```python
from build123d import *

# Parameters (mm, degrees)
SKETCH_1_R                  = 3
EXTRUDE_1_DEPTH             = 9
SKETCH_2_R                  = 6
EXTRUDE_2_DEPTH             = 1.2
DOME_1_FACE_RADIUS          = 6
DOME_1_HEIGHT               = 3
MIRROR_1_COPY_1_FACE_RADIUS = 6
MIRROR_1_COPY_1_HEIGHT      = 3


with BuildPart() as part:
    # Эскиз1 → Бобышка-Вытянуть1 (new, symmetric)
    with BuildSketch(Plane(origin=(0, 0, 0), x_dir=(1, 0, 0), z_dir=(0, 1, 0))):
        with Locations(Location((0, 0, 0), (0, 0, 270))):
            Circle(SKETCH_1_R)
    extrude(amount=EXTRUDE_1_DEPTH, both=True)

    # Эскиз2 → Бобышка-Вытянуть2 (add)
    with BuildSketch(Plane(origin=(0, 9, 0), x_dir=(1, 0, 0), z_dir=(0, 1, 0))):
        with Locations(Location((0, 0, 0), (0, 0, 270))):
            Circle(SKETCH_2_R)
    extrude_2 = extrude(amount=EXTRUDE_2_DEPTH)

    # Купол1: a dome of height H over a round flat face of radius A is a cap of a sphere of radius (A * A + H * H) / (2 * H)
    dome_1_r = (DOME_1_FACE_RADIUS * DOME_1_FACE_RADIUS + DOME_1_HEIGHT * DOME_1_HEIGHT) / (2 * DOME_1_HEIGHT)
    dome_1_base = Plane((0, 10.2, 0), z_dir=(0, 1, 0))
    with Locations(dome_1_base.offset(DOME_1_HEIGHT - dome_1_r)):
        dome_1_ball = Sphere(dome_1_r, mode=Mode.PRIVATE)
    add(split(dome_1_ball, bisect_by=dome_1_base, keep=Keep.TOP, mode=Mode.PRIVATE))

    # Зеркальное отражение1: Бобышка-Вытянуть2 across plane
    add(extrude_2.mirror(Plane.ZX))

    # Зеркальное отражение1 copy 1: a dome of height H over a round flat face of radius A is a cap of a sphere of radius (A * A + H * H) / (2 * H)
    mirror_1_copy_1_r = (MIRROR_1_COPY_1_FACE_RADIUS * MIRROR_1_COPY_1_FACE_RADIUS + MIRROR_1_COPY_1_HEIGHT * MIRROR_1_COPY_1_HEIGHT) / (2 * MIRROR_1_COPY_1_HEIGHT)
    mirror_1_copy_1_base = Plane((0, -10.2, 0), z_dir=(0, -1, 0))
    with Locations(mirror_1_copy_1_base.offset(MIRROR_1_COPY_1_HEIGHT - mirror_1_copy_1_r)):
        mirror_1_copy_1_ball = Sphere(mirror_1_copy_1_r, mode=Mode.PRIVATE)
    add(split(mirror_1_copy_1_ball, bisect_by=mirror_1_copy_1_base, keep=Keep.TOP, mode=Mode.PRIVATE))


solid = part.part
```
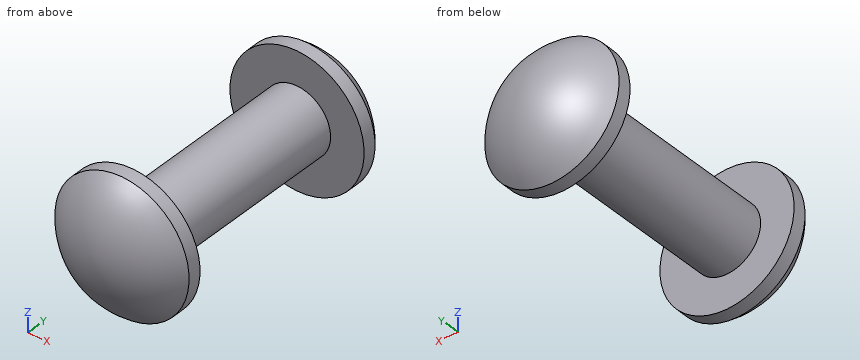
Work out the finished part from the listing and answer in its coordinate system (mm). Round coordinates to 2 decimals unless told otherwise and drop trailing zeros. Write each loop counter-clockwise with the first axis right and the second up, starting at its lowest first coordinate (ties: lowest second). Pieces come first, ordered by that corner, then holes. Notation, with made-up numbers: (62, -24.75) - (82, -24.75) arc R11 cw to (82, -13.75) - close; hole circle Ø5 at (85, 85). An arc over 180 degrees is marked (long way). Return JSON: item names as keys, results as strings. Group by question number.
Q1. Find the intervals of material crossed by L1, parallel to X at y = 5.5, z = 0; L2, parallel to Y at x = 4, z = -3.5; L3, parallel to Y at x = -3.5, z = 0.75, in increasing order.
Q2. The part is cut by section A-A on z = 0. Write down the section's boundary in (x, y), then the cut area to 3 significant figures.
Q3. The part is cut by section B-B on x = 0. Write down the section's boundary in (y, z), then the cut area to 3 significant figures.
Q4. Each of these flat-tipped pins is pushed along its axis until it touches: pin 1 Ø6 at (x, z) = (1, 0.5) entering from +Y; pin 2 Ø5 at (y, z) = (2, -2.5) entering from -X; pin 3 Ø2 at (x, z) = (-1.5, 0) entering from -Y; pin 4 Ø1.5 at (x, y) = (-1.5, 8) entering from -Z. Where does it stop, or does it pass through?
Q5. The part is cut by section D-D on y = 5. Write down the section's boundary in (x, z), then the cut area to 3 significant figures.
Q6. The part is cut by section C-C on z = 4.75. Write down the section's boundary in (x, y).
Solved:
{
 "1": {"L1": "-3 to 3", "L2": "-10.99 to -9, 9 to 10.99", "L3": "-12.29 to -9, 9 to 12.29"},
 "2": {"outline": "(-6, -10.2) arc R7.5 ccw to (6, -10.2) - (6, -9) - (3, -9) - (3, 9) - (6, 9) - (6, 10.2) arc R7.5 ccw to (-6, 10.2) - (-6, 9) - (-3, 9) - (-3, -9) - (-6, -9) - close", "area": "187 mm²"},
 "3": {"outline": "(-10.2, -6) - (-9, -6) - (-9, -3) - (9, -3) - (9, -6) - (10.2, -6) arc R7.5 ccw to (10.2, 6) - (9, 6) - (9, 3) - (-9, 3) - (-9, 6) - (-10.2, 6) arc R7.5 ccw to start", "area": "187 mm²"},
 "4": {"pin 1": "y = 13.2", "pin 2": "x = -3", "pin 3": "y = -13.18", "pin 4": "z = -2.9"},
 "5": {"outline": "circle Ø6 at (0, 0)", "area": "28.3 mm²"},
 "6": {"outline": "(-3.67, -10.2) arc R5.8 ccw to (3.67, -10.2) - (3.67, -9) - (-3.67, -9) - close; (-3.67, 9) - (3.67, 9) - (3.67, 10.2) arc R5.8 ccw to (-3.67, 10.2) - close"}
}
